For this review, use the dimensioned drawing (mm, ordinates from the lowest corner) and the shaded views. Give positions to 0.01 mm unless a question says otherwise; leave off trailing zeros. Loops run counter-clockwise (first coordinate to the right, second up) from the corner with the lowest first, then second, coordinate; pieces in that order, holes last. Notation, with made-up numbers: (62.5, 78) -> (106.5, 78) arc R20 ccw to (106.5, 111) -> close; hole circle Ø3 at (5, 1). An arc over 180 degrees is marked (long way). Write each question's results on one line, items separated by ' | '. Start each with the question number.
Q1. Wall thickness on L1, parallel to X at y = 63, z = 19; L2, parallel to Y at x = 88.9, z = 13.5; L3, parallel to Y at x = 88, z = 15: over which ranges is each line inside the solid? List them lowest first. Write a range as [from, to].
Q2. Insertion check: pin 1 Ø1 at (x, y) = (79, 31) entering from +Z; pin 2 Ø1.5 at (x, z) = (84, 66.5) entering from +Y; pin 3 Ø1 at (x, y) = (177.5, 24.5) entering from +Z. Each pin has a flat end and moves straight along its axis. Give the tip position at first contact, or say it passes through.
Q3. We need section B-B (x = 88.9). Write out the cut boundary in (y, z).
Q4. We need section A-A (y = 63.5). Write out the cut boundary in (x, z).
Q5. We need section C-C (z = 83). Write out the cut boundary in (x, y).
Q6. We need section D-D (y = 22). Write out the cut boundary in (x, z).
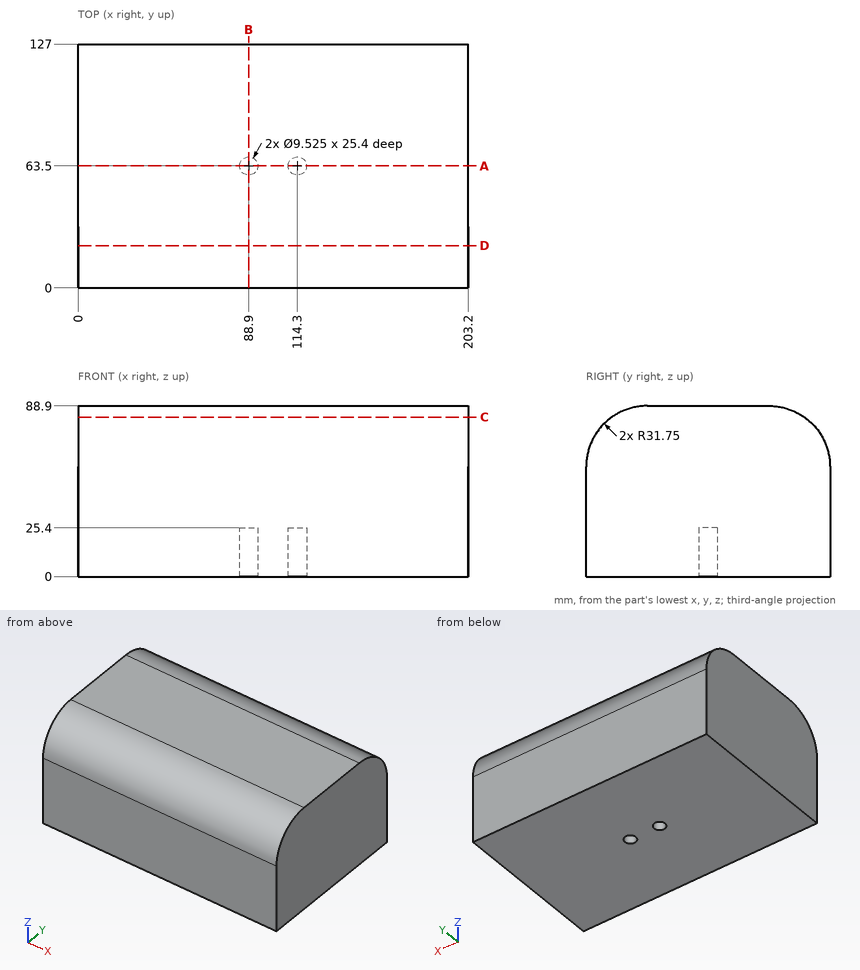
Output:
1) L1: [0, 84.16], [93.64, 109.56], [119.04, 203.2] | L2: [0, 58.74], [68.26, 127] | L3: [0, 58.82], [68.18, 127]
2) pin 1: z = 88.9 | pin 2: y = 125.81 | pin 3: z = 88.17
3) outline: (0, 0) -> (58.74, 0) -> (58.74, 25.4) -> (68.26, 25.4) -> (68.26, 0) -> (127, 0) -> (127, 57.15) arc R31.75 ccw to (95.25, 88.9) -> (31.75, 88.9) arc R31.75 ccw to (0, 57.15) -> close
4) outline: (0, 0) -> (84.14, 0) -> (84.14, 25.4) -> (93.66, 25.4) -> (93.66, 0) -> (109.54, 0) -> (109.54, 25.4) -> (119.06, 25.4) -> (119.06, 0) -> (203.2, 0) -> (203.2, 88.9) -> (0, 88.9) -> close
5) outline: (0, 13.32) -> (203.2, 13.32) -> (203.2, 113.68) -> (0, 113.68) -> close
6) outline: (0, 0) -> (203.2, 0) -> (203.2, 87.37) -> (0, 87.37) -> close
